Verification items for this drawing (mm, ordinates from the low corner). Round coordinates to 2 decimals unless told otherwise and drop trailing zeros. Write each loop counter-clockwise with the first axis right and the second up, starting at its lowest first coordinate (ties: lowest second). Pieces come first, ordered by that corner, then holes. Notation, with made-up numbers: (38.25, 47) -> (84.25, 47) arc R6 cw to (84.25, 54) -> close; hole circle Ø7 at (5, 77). An arc over 180 degrees is marked (long way). Put each result on its own line as item: value. Start each with the question number.
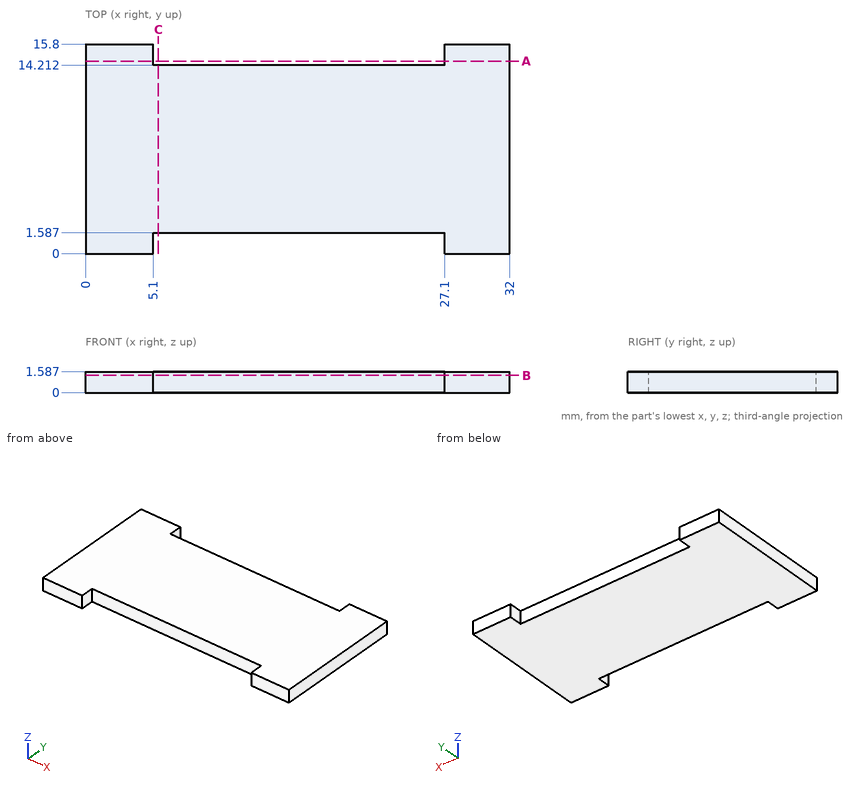
1. Section check C-C, the plane x = 5.5. Enter the section's corners in (y, z).
2. Section check A-A, the plane y = 14.5. Enter the section's corners in (x, z).
3. Gauge pin test, flat end, axial feed: P1, Ø0.5, axis at x = 21.5, z = 0.5, coming from the +Y side. Record the tip position at first contact, or that the pin passes through.
4. Section check B-B, the plane z = 1.3. Enter the section's corners in (x, y), then the cut area to 3 significant figures.
5. Material ranges on L1, parallel to X at y = 14.25, z = 0.4; L2, parallel to Y at x = 26.5, z = 0.4, recorded low to high. Write a range as [from, to].
Reply:
1. outline: (1.59, 0) -> (14.21, 0) -> (14.21, 1.59) -> (1.59, 1.59) -> close
2. outline: (0, 0) -> (5.1, 0) -> (5.1, 1.59) -> (0, 1.59) -> close; (27.1, 0) -> (32, 0) -> (32, 1.59) -> (27.1, 1.59) -> close
3. P1: stops at y = 14.21
4. outline: (0, 0) -> (5.1, 0) -> (5.1, 1.59) -> (27.1, 1.59) -> (27.1, 0) -> (32, 0) -> (32, 15.8) -> (27.1, 15.8) -> (27.1, 14.21) -> (5.1, 14.21) -> (5.1, 15.8) -> (0, 15.8) -> close
4. area: 436 mm2
5. L1: x = [0, 5.1], [27.1, 32]
5. L2: y = [1.59, 14.21]
